Check sheet for the modelled part. Datum: model origin and axes. Units: mm. A direction names the side the tool comes from. Give positions to 0.01 mm unless a question says otherwise; leave off trailing zeros. Loops run counter-clockwise (first coordinate to the right, second up) from the corner with the lowest first, then second, coordinate; pieces in that order, holes last. Notation, with made-up numbers: (88.25, 12.25) - (132.25, 12.25) arc R23 cw to (132.25, 24.25) - close; hole circle Ø4 at (-7, 29.25). An arc over 180 degrees is marked (long way). Answer in a Markdown table with one row per item. Add a question column.
(1) Sectioned sample at B-B on x = 0. Enter the section's corners in (y, z).
(2) Set-up check for faces 1 (the face through (0, -6, 21)), 2 (the face through (-4.092, 10.905, 13.601)), 3 (the face through (-2, -2, 9)): record each of +Z, -Z, +X, -X, +Y, -Y from which the full face is reachable in a straight line by a thin tool's end or side.
(3) Sectioned sample at A-A on y = 0. Enter the section's corners in (x, z).
(4) Thickness scan on L1, parallel to Y at x = 0, z = 20.75; L2, parallel to Y at x = 0, z = 1.75; L3, parallel to X at y = -7.5, z = 14. Record the ranges inside material, lowest first.
(5) Go/stop test with flat-tipped pins: P1, Ø1, axis at x = -6, z = 13.5, coming from the +Y side; P2, Ø6, axis at x = 0, y = 0, coming from the -Z side; P3, Ø12, axis at x = -9, z = 4.5, coming from the +Y side. Record where each tip stops, or that it passes through.
(6) Draft check along Z on faces 4 (the face through (3, 0, 25)), 5 (the face through (-6, -7.8, 13)), 6 (the face through (-4, -2, 3)). Enter one of: released by +Z, released by -Z, zero draft, split by the parting line, or undercut.
(7) Sectioned sample at C-C on z = 13. Enter the section's corners in (x, y).
from build123d import *

# Parameters (mm, degrees)
F4_R      = 1.55
F5_DEPTH  = 4
F7_R      = 1.6
F8_DEPTH  = 20.8
F10_R     = 2
F11_DEPTH = 3


with BuildPart() as f1:
    # F0 (on Front) → F1 (revolve)
    with BuildSketch(Plane.XZ):
        with BuildLine():
            Line((10, 3), (10, 0.190525))
            ThreePointArc((10, 0.190525), (11.5, 0), (13, 0.190525))
            Line((13, 0.190525), (13, 25))
            Line((13, 25), (2.5, 25))
            Line((2.5, 25), (2.5, 9))
            Line((2.5, 9), (4.25, 9))
            Line((4.25, 9), (4.25, 3))
            Line((4.25, 3), (10, 3))
        make_face()
    revolve(axis=Axis((0, 0, 12.5), (0, 0, 1)))

    # F4 (on offset) → F5 (cut)
    with BuildSketch(Plane.XY.offset(25)):
        with Locations((0, -6.5)):
            Circle(F4_R)
    extrude(amount=-F5_DEPTH, mode=Mode.SUBTRACT)

    # F7 (on offset) → F8 (cut)
    with BuildSketch(Plane.XZ.offset(-13)):
        with Locations((-6, 13)):
            Circle(F7_R)
    extrude(amount=F8_DEPTH, mode=Mode.SUBTRACT)

    # F10 (on offset) → F11 (cut)
    with BuildSketch(Plane.XZ.offset(-10)):
        with Locations((-6, 13)):
            Circle(F10_R)
    extrude(amount=-F11_DEPTH, mode=Mode.SUBTRACT)


solid = f1.part
Reply:
| question | item | result |
|---|---|---|
| 1 | outline | (-13, 0.19) arc R6 ccw to (-10, 0.19) - (-10, 3) - (-4.25, 3) - (-4.25, 9) - (-2.5, 9) - (-2.5, 25) - (-4.95, 25) - (-4.95, 21) - (-8.05, 21) - (-8.05, 25) - (-13, 25) - close; (2.5, 9) - (4.25, 9) - (4.25, 3) - (10, 3) - (10, 0.19) arc R6 ccw to (13, 0.19) - (13, 25) - (2.5, 25) - close |
| 2 | face 1 | +Z |
| 2 | face 2 | +Y |
| 2 | face 3 | -Z |
| 3 | outline | (-13, 0.19) arc R6 ccw to (-10, 0.19) - (-10, 3) - (-4.25, 3) - (-4.25, 9) - (-2.5, 9) - (-2.5, 25) - (-13, 25) - close; (2.5, 9) - (4.25, 9) - (4.25, 3) - (10, 3) - (10, 0.19) arc R6 ccw to (13, 0.19) - (13, 25) - (2.5, 25) - close; hole circle Ø3.2 at (-6, 13) |
| 4 | L1 | -13 to -2.5, 2.5 to 13 |
| 4 | L2 | -13 to -10, 10 to 13 |
| 4 | L3 | -10.62 to -7.25, -4.75 to 10.62 |
| 5 | P1 | y = -7.8 |
| 5 | P2 | z = 9 |
| 5 | P3 | y = 12.65 |
| 6 | face 4 | released by +Z |
| 6 | face 5 | undercut |
| 6 | face 6 | released by -Z |
| 7 | outline | (-8, 10) - (-8, 10.25) arc R13 ccw (long way) to (-4, 12.37) - (-4, 10) - (-4.4, 10) - (-4.4, -7.8) - (-7.6, -7.8) - (-7.6, 10) - close; hole circle Ø5 at (0, 0) |
